Verification items for this drawing (mm, ordinates from the low corner). A direction names the side the tool comes from. Round coordinates to 2 decimals unless told otherwise and drop trailing zeros. Order: outer loops, then holes, each group sorted by start corner. A loop starts at its lowest first (then second) coordinate and runs counter-clockwise, first axis right, second up. Notation, with made-up numbers: (-14.75, 26.25) -> (37.25, 26.25) arc R18 cw to (37.25, 41.25) -> close; hole circle Ø7 at (78, -36). An arc over 180 degrees is marked (long way). Return JSON: item names as keys, results as strings. Group by question number.
Item 1: Sectioned sample at B-B on x = 21. Give the number of separate pieces and of enclosed holes in the cut face, plus the area to 3 significant figures.
Item 2: Draft check along Z on the marked faces 1, 2 and 3. Enter one of: pulls with the +Z half, pulls with the -Z half, needs draft (parallel to the pull), parting line crosses it, or undercut.
Item 3: Depth check by flat-ended pin: pin 1 Ø8 at (x, z) = (37.5, 45.5) entering from -Y; pin 2 Ø4 at (y, z) = (2, 20) entering from -X; pin 3 Ø8 at (x, y) = (16, 6.5) entering from -Z. Enter the tip coordinate at first touch or a pass-through.
Item 4: Scan lines: probe 1 along Z at (x, y) = (19.82, 9.75); probe 2 along Z at (x, y) = (17.5, 13.25); probe 3 along X at (y, z) = (1.25, 36.5). Record each from-to range of solid material in increasing order. Write a range as from..to.
Item 5: Sectioned sample at A-A on y = 4.5. Record the cut outline in (x, z), plus the area to 3 significant figures.
Item 6: Access from +Z, -Z, +X, -X, +Y, -Y to the whole of each face (thin tool, end or side, straight path). Record for the marked faces 4, 5 and 6.
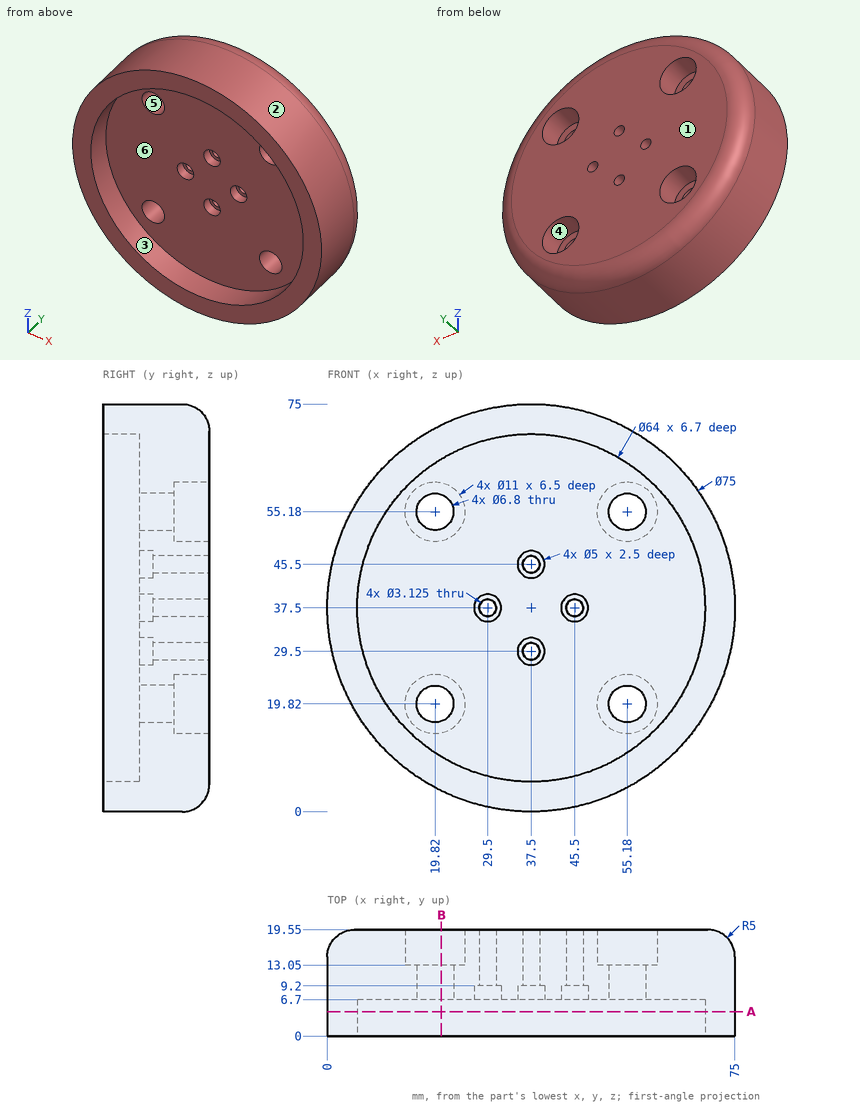
Recorded:
{
 "1": {"separate pieces": "3", "enclosed holes": "0", "area": "717 mm²"},
 "2": {"face 1": "needs draft", "face 2": "parting line crosses it", "face 3": "undercut"},
 "3": {"pin 1": "y = 6.7", "pin 2": "x = 3.35", "pin 3": "z = 4.33"},
 "4": {"probe 1": "4.43..16.42, 23.22..51.78, 58.58..70.57", "probe 2": "5.78..14.83, 24.81..50.19, 60.17..69.22", "probe 3": "0.01..5.52, 69.48..74.99"},
 "5": {"outline": "circle Ø75 at (37.5, 37.5); hole circle Ø64 at (37.5, 37.5)", "area": "1,200 mm²"},
 "6": {"face 4": "+Y", "face 5": "+Y, -Y", "face 6": "-Y"}
}
